Source: CAD feature listing. Evaluate the final solid. Frame: model axes, mm. Face numbers are marked on the shaded views. A direction names the side the tool comes from. Give positions to 0.01 mm unless a question says otherwise; leave off trailing zeros. Loops run counter-clockwise (first coordinate to the right, second up) from the corner with the lowest first, then second, coordinate; pieces in that order, holes last. Notation, with made-up numbers: M -37,-15.5 L -17,-15.5 A16 cw -17,-2.5 Z; hole C 89.5,18 d10. An arc over 180 degrees is marked long. Answer in a Markdown table with one row per item.
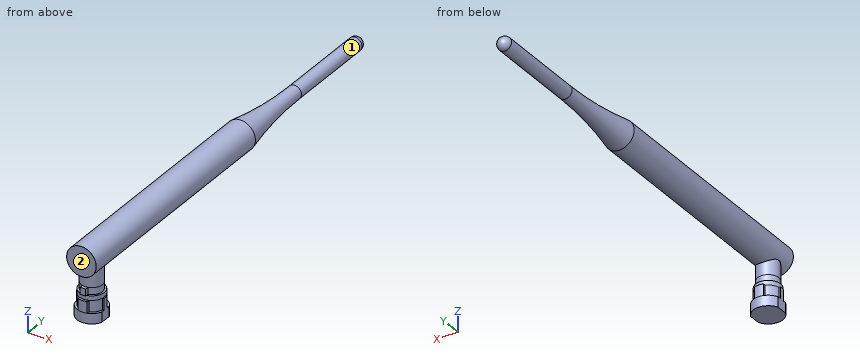
```python
from build123d import *

# Parameters (mm, degrees)
BOSS_EXTRUDE1_DEPTH      = 4.5
BOSS_EXTRUDE2_DEPTH      = 5
SKETCH3_R                = 5.5
BOSS_EXTRUDE3_DEPTH      = 2
BOSS_EXTRUDE4_DEPTH      = 3
SKETCH5_R                = 4.65
BOSS_EXTRUDE5_DEPTH      = 12
BOSS_EXTRUDE6_DEPTH      = 100
BOSS_EXTRUDE6_DEPTH_BACK = 7
SKETCH6_R                = 6.5
SKETCH7_R                = 3
BOSS_EXTRUDE7_DEPTH      = 80
FILLET1_R                = 190
FILLET2_R                = 3


with BuildPart() as part:
    # Sketch1 → Boss-Extrude1 (new body)
    with BuildSketch(Plane.XY):
        with BuildLine():
            Line((-6, 2.5), (-6, -2.5))
            ThreePointArc((-6, -2.5), (0, -6.5), (6, -2.5))
            Line((6, -2.5), (6, 2.5))
            ThreePointArc((6, 2.5), (0, 6.5), (-6, 2.5))
        make_face()
    extrude(amount=BOSS_EXTRUDE1_DEPTH)

    # Sketch2 → Boss-Extrude2 (add)
    with BuildSketch(Plane.XY.offset(4.5)):
        with BuildLine():
            ThreePointArc((2, 6.184658438), (0, 6.5), (-2, 6.184658438))
            Line((-2, 6.184658438), (-2, 5.123475383))
            ThreePointArc((-2, 5.123475383), (-4.239291123, 3.504056332), (-5.408326913, 1))
            Line((-5.408326913, 1), (-6, 1))
            Line((-6, 1), (-6, -1))
            Line((-6, -1), (-5.408326913, -1))
            ThreePointArc((-5.408326913, -1), (-4.239291123, -3.504056332), (-2, -5.123475383))
            Line((-2, -5.123475383), (-2, -6.184658438))
            ThreePointArc((-2, -6.184658438), (0, -6.5), (2, -6.184658438))
            Line((2, -6.184658438), (2, -5.123475383))
            ThreePointArc((2, -5.123475383), (4.239291123, -3.504056332), (5.408326913, -1))
            Line((5.408326913, -1), (6, -1))
            Line((6, -1), (6, 1))
            Line((6, 1), (5.408326913, 1))
            ThreePointArc((5.408326913, 1), (4.239291123, 3.504056332), (2, 5.123475383))
            Line((2, 5.123475383), (2, 6.184658438))
        make_face()
    extrude(amount=BOSS_EXTRUDE2_DEPTH)

    # Sketch3 → Boss-Extrude3 (add)
    with BuildSketch(Plane.XY.offset(9.5)):
        with Locations(Location((0, 0, 0), (0, 0, 169.524318304))):
            Circle(SKETCH3_R)
    extrude(amount=BOSS_EXTRUDE3_DEPTH)

    # Sketch4 → Boss-Extrude4 (add)
    with BuildSketch(Plane.XY.offset(11.5)):
        with BuildLine():
            Line((-1.2, -4.49249374), (-1.2, -5.99249374))
            Line((-1.2, -5.99249374), (1.2, -5.99249374))
            Line((1.2, -5.99249374), (1.2, -4.49249374))
            ThreePointArc((1.2, -4.49249374), (0, 4.65), (-1.2, -4.49249374))
        make_face()
    extrude(amount=BOSS_EXTRUDE4_DEPTH)

    # Sketch5 → Boss-Extrude5 (add)
    with BuildSketch(Plane.XY.offset(14.5)):
        with Locations(Location((0, 0, 0), (0, 0, 255.044751683))):
            Circle(SKETCH5_R)
    extrude(amount=BOSS_EXTRUDE5_DEPTH)

    # Sketch6 → Boss-Extrude6 (add, two sides: drawn at the far end of the back side and taken through both)
    with BuildSketch(Plane(origin=(0, 0, 0), x_dir=(1, 0, 0), z_dir=(0, 1, 0)).offset(-BOSS_EXTRUDE6_DEPTH_BACK)):
        with Locations(Location((0, -26.5, 0), (0, 0, 270))):
            Circle(SKETCH6_R)
    extrude(amount=BOSS_EXTRUDE6_DEPTH + BOSS_EXTRUDE6_DEPTH_BACK)

    # Sketch7 → Boss-Extrude7 (add)
    with BuildSketch(Plane(origin=(0, 100, 0), x_dir=(1, 0, 0), z_dir=(0, 1, 0))):
        with Locations(Location((0, -26.5, 0), (0, 0, 270))):
            Circle(SKETCH7_R)
    extrude(amount=BOSS_EXTRUDE7_DEPTH)

    # Fillet1
    # the kernel refuses this fillet: 190 mm, written as the material it adds along each edge
    with BuildSketch(Plane(origin=(0, 100, 26.5), x_dir=(0, 0, 1), z_dir=(-1, 0, 0))) as fillet1_piece_1:
        with BuildLine():
            CenterArc((193, 36.300826437), FILLET1_R, 180, 11.014474836)
            Line((3, 36.300826437), (0, 36.300826437))
            Line((0, 36.300826437), (0, 0))
            Line((0, 0), (3, -3.8))
            ThreePointArc((3, -3.8), (4.75, -3.8), (2.77, -0.726016529))
            Line((2.77, -0.726016529), (6.5, 0))
        make_face()
    revolve(axis=Axis((0, 100, 26.5), (0, 1, 0)))

    # Fillet2
    fillet2_edges = [part.edges().sort_by_distance(p)[0] for p in [
        (0, 180, 23.5),
    ]]
    fillet(fillet2_edges, radius=FILLET2_R)


solid = part.part
```
Q1. Contact query for flat-ended pins moving along their axis: pin 1 Ø2 at (x, z) = (-5, 11) entering from -Y; pin 2 Ø1.1 at (x, y) = (1, -6) entering from +Z; pin 3 Ø4.5 at (x, y) = (5, -4) entering from +Z. Output: stop coordinate, or through.
Values follow:
| item | result |
|---|---|
| pin 1 | y = -3.77 |
| pin 2 | z = 32.98 |
| pin 3 | z = 32.39 |
Q2. Reachability of the marked faces 1 and 2 from +Z, -Z, +X, -X, +Y, -Y: full face, straight path, thin tool, end or side. Return the list, or none.
Values follow:
| item | result |
|---|---|
| face 1 | +Y |
| face 2 | +Z, -Z, +X, -X, -Y |
Q3. Section query C-C (z = 18). Output: boundary loops of the cut face in (x, y).
Values follow:
| item | result |
|---|---|
| outline | C 0,0 d9.3 |
Q4. Section query A-A (z = 26.5). Output: boundary loops of the cut face in (x, y).
Values follow:
| item | result |
|---|---|
| outline | M -6.5,-7 L 6.5,-7 L 6.5,100 A190 cw 3,136.3 L 3,177 A3 ccw -3,177 L -3,136.3 A190 cw -6.5,100 Z |
Q5. Section query B-B (y = 75). Output: boundary loops of the cut face in (x, z), plus the area to 3 significant figures.
Values follow:
| item | result |
|---|---|
| outline | C 0,26.5 d13 |
| area | 133 mm^2 |
Q6. Ray query, probe 1 along X at (y, z) = (10.5, 22.5); probe 2 along Y at (x, z) = (0.25, 10.5); probe 3 along Z at (x, y) = (-0.25, 171). Return the intervals inside material, ascending. Write a range as from..to.
Values follow:
| item | result |
|---|---|
| probe 1 | -5.12..5.12 |
| probe 2 | -5.49..5.49 |
| probe 3 | 23.51..29.49 |
